from build123d import *

# Parameters (mm, degrees)
F0_W     = 525
F0_H     = 70
F1_DEPTH = 45
F2_R     = 11
F3_DEPTH = 45.001
F4_R     = 11
F5_DEPTH = 45.001


with BuildPart() as f1:
    # F0 (on Front) → F1 (new body)
    with BuildSketch(Plane.XZ):
        with Locations((-262.5, -35)):
            Rectangle(F0_W, F0_H)
    extrude(amount=F1_DEPTH)

    # F2 (on face) → F3 (cut, through all)
    with BuildSketch(Plane(origin=(0, 0, 0), x_dir=(-1, 0, 0), z_dir=(0, 1, 0))):
        with Locations((495, -24)):
            Circle(F2_R)
    extrude(amount=-F3_DEPTH, mode=Mode.SUBTRACT)

    # F4 (on face) → F5 (cut, through all)
    with BuildSketch(Plane(origin=(0, 0, 0), x_dir=(-1, 0, 0), z_dir=(0, 1, 0))):
        with Locations((47, -24)):
            Circle(F4_R)
    extrude(amount=-F5_DEPTH, mode=Mode.SUBTRACT)


solid = f1.part
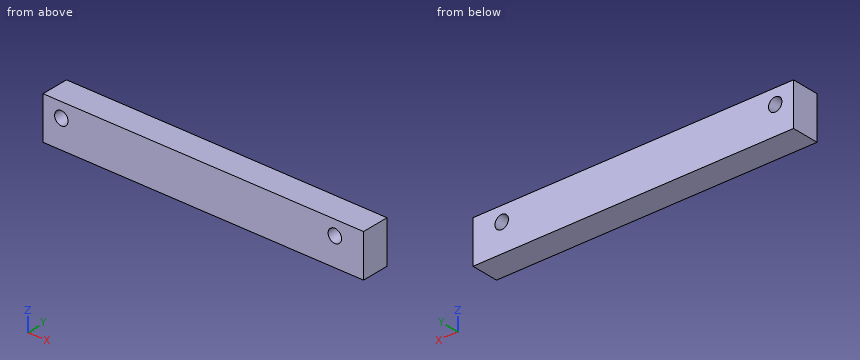
Can you work these out from the model? Positions are in its coordinate system, mm. Coordinates: 2 decimals unless noted, no trailing zeros. Write each loop counter-clockwise with the first axis right and the second up, starting at its lowest first coordinate (ties: lowest second). Pieces come first, ordered by that corner, then holes.
Q1. Imagine slicing it at B-B, the plane x = -495. List the corners of the cut face in (y, z) for me, plus the area to 3 significant figures.
Results found:
outline: (-45, -70) - (0, -70) - (0, -35) - (-45, -35) - close; (-45, -13) - (0, -13) - (0, 0) - (-45, 0) - close
area: 2,160 mm2
Q2. Please list where these lines run through material, in increasing order: L1, parallel to Z at x = -47, y = -31; L2, parallel to X at y = -2, z = -19.5; L3, parallel to X at y = -32, z = -20.
Results found:
L1: z = -70 to -35, -13 to 0
L2: x = -525 to -505.04, -484.96 to -57.04, -36.96 to 0
L3: x = -525 to -505.25, -484.75 to -57.25, -36.75 to 0
Q3. Imagine slicing it at A-A, the plane z = -24. List the corners of the cut face in (x, y) for me.
Results found:
outline: (-525, -45) - (-506, -45) - (-506, 0) - (-525, 0) - close; (-484, -45) - (-58, -45) - (-58, 0) - (-484, 0) - close; (-36, -45) - (0, -45) - (0, 0) - (-36, 0) - close
Q4. Imagine slicing it at C-C, the plane y = -30. List the corners of the cut face in (x, z) for me, plus the area to 3 significant figures.
Results found:
outline: (-525, -70) - (0, -70) - (0, 0) - (-525, 0) - close; hole circle Ø22 at (-495, -24); hole circle Ø22 at (-47, -24)
area: 36,000 mm2
